For this review, use the dimensioned drawing (mm, ordinates from the lowest corner) and the shaded views. Coordinates: 2 decimals unless noted, no trailing zeros. Loops run counter-clockwise (first coordinate to the right, second up) from the corner with the lowest first, then second, coordinate; pieces in that order, holes last.
1. Clearance check with flat-ended pins moving along their axes: P1, Ø6, axis at x = 10.5, z = 34.5, coming from the +Y side; P2, Ø12, axis at y = 17.5, z = 27, coming from the +X side; P3, Ø1, axis at y = 17.5, z = 32.5, coming from the +X side. State where each tip first meets the part, or that it passes through.
2. Take a section at A-A, the plane z = 31.5. State the section outline as (x, y) points (3 decimals).
3. To check wall thickness, follow probe 1 along Y at (x, z) = (13.75, 7); probe 2 along X at (y, z) = (6, 10); probe 3 along Y at (x, z) = (14.75, 7). State the ranges of each line that lie inside material, in increasing order.
4. Take a section at B-B, the plane z = 15. State the section outline as (x, y) points (3 decimals), then the cut area to 3 significant figures.
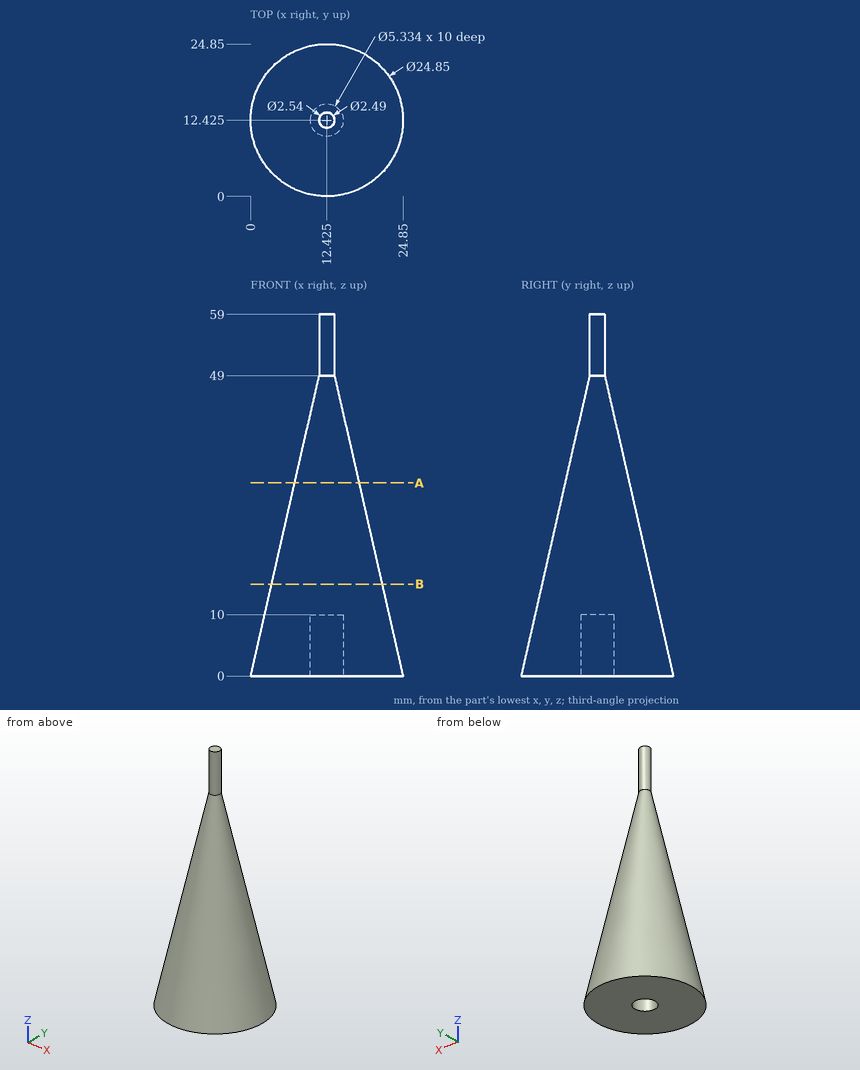
Results list:
1. P1: stops at y = 17.56
1. P2: stops at x = 19.64
1. P3: stops at x = 14.5
2. outline: circle Ø10.476 at (12.425, 12.425)
3. probe 1: y = 1.68 to 10.11, 14.74 to 23.17
3. probe 2: x = 4.58 to 20.27
3. probe 3: y = 1.85 to 11.12, 13.73 to 23
4. outline: circle Ø18.005 at (12.425, 12.425)
4. area: 255 mm2
